Answer from the drawing. Dimensions are ordinates in mm from the lowest x, y and z of the part. A direction names the side the tool comes from. Give positions to 0.01 mm unless a question says otherwise; leave off trailing zeros. Order: outer loops, then holes, each group sorted by start corner. A loop starts at its lowest first (then second) coordinate and runs counter-clockwise, first axis right, second up. Notation, with made-up numbers: (-21, 49.25) - (-15, 49.25) arc R28 cw to (-15, 84.25) - close; hole circle Ø2 at (48.25, 21). An arc over 180 degrees is marked (long way). Answer in a Markdown table with one row per item. Add a question column.
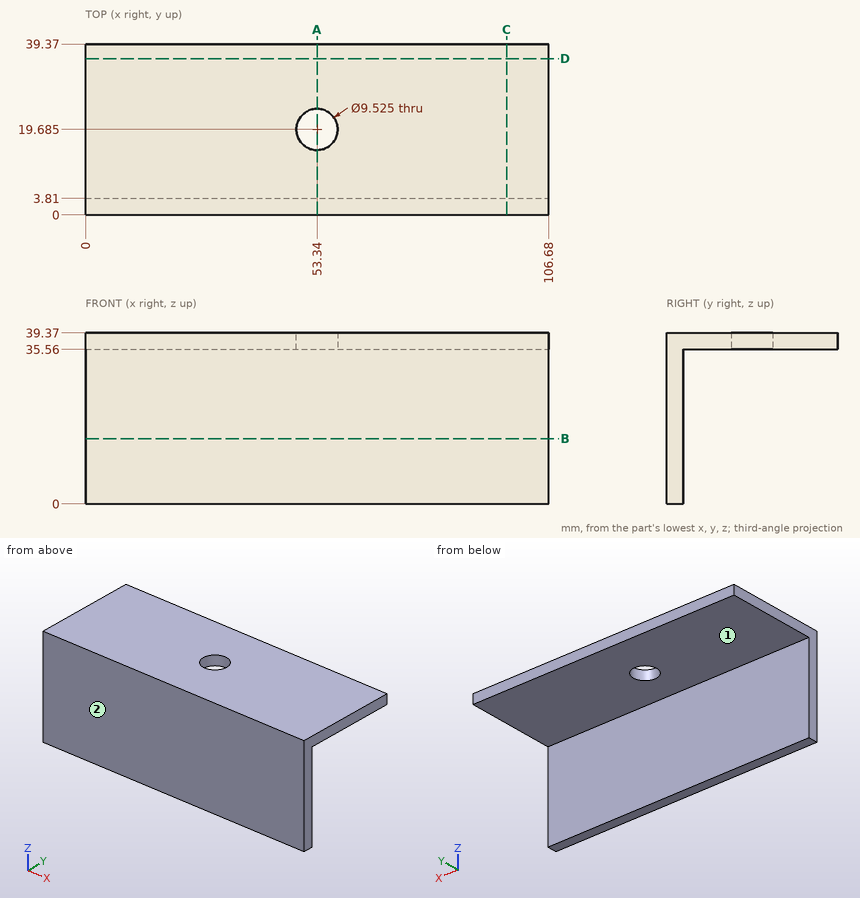
(1) For the marked faces 1 and 2, determine the directions among +Z, -Z, +X, -X, +Y, -Y from which every point of the face is accessible in a straight line to the end or side of a thin tool.
(2) Each of these flat-tipped pins is pushed along its axis until it touches: P1, Ø10.5, axis at x = 59, z = 18.5, coming from the +Y side; P2, Ø10.5, axis at x = 28, y = 14.5, coming from the -Z side; P3, Ø6, axis at x = 88.5, z = 25.5, coming from the -Y side. Where does it stop, or does it pass through?
(3) Find section A-A, the plane x = 53.34. Write down the section's boundary in (y, z).
(4) Find section C-C, the plane x = 97. Write down the section's boundary in (y, z).
(5) Straight lines are drawn through the part: line 1 (Y direction, x = 53.34, z = 36.45); line 2 (Y direction, x = 29.5, z = 26.5); line 3 (Z direction, x = 70, y = 35). For each, find the intervals that lie inside material, in ascending order.
(6) Find section B-B, the plane z = 15. Write down the section's boundary in (x, y), plus the area to 3 significant figures.
(7) Find section D-D, the plane y = 36. Write down the section's boundary in (x, z), plus the area to 3 significant figures.
Answer key:
| question | item | result |
|---|---|---|
| 1 | face 1 | -Z, +X, -X, +Y |
| 1 | face 2 | +Z, -Z, +X, -X, -Y |
| 2 | P1 | y = 3.81 |
| 2 | P2 | z = 35.56 |
| 2 | P3 | y = 0 |
| 3 | outline | (0, 0) - (3.81, 0) - (3.81, 35.56) - (14.92, 35.56) - (14.92, 39.37) - (0, 39.37) - close; (24.45, 35.56) - (39.37, 35.56) - (39.37, 39.37) - (24.45, 39.37) - close |
| 4 | outline | (0, 0) - (3.81, 0) - (3.81, 35.56) - (39.37, 35.56) - (39.37, 39.37) - (0, 39.37) - close |
| 5 | line 1 | 0 to 14.92, 24.45 to 39.37 |
| 5 | line 2 | 0 to 3.81 |
| 5 | line 3 | 35.56 to 39.37 |
| 6 | outline | (0, 0) - (106.68, 0) - (106.68, 3.81) - (0, 3.81) - close |
| 6 | area | 406 mm² |
| 7 | outline | (0, 35.56) - (106.68, 35.56) - (106.68, 39.37) - (0, 39.37) - close |
| 7 | area | 406 mm² |
